```python
from build123d import *

# Parameters (mm, degrees)
EXTRUDE_1_DEPTH     = 12
EXTRUDE_3_DEPTH     = 6
SKETCH_4_R          = 2
EXTRUDE_4_DEPTH     = 4
CUT_EXTRUDE_2_DEPTH = 29.284271247


with BuildPart() as part:
    # 草图1 → 凸台-拉伸1 (new body)
    with BuildSketch(Plane.XY):
        Polygon((-11, 12.536842105), (-16, 12.536842105), (-16, 14.536842105), (-11, 14.536842105), (-11, 16.036842105), (11, 16.036842105), (11, 14.536842105), (16, 14.536842105), (16, 12.536842105), (11, 12.536842105), (11, -5.463157895), (-11, -5.463157895), align=None)
    extrude(amount=EXTRUDE_1_DEPTH)

    # 草图2 → 凸台-拉伸3 (add)
    with BuildSketch(Plane(origin=(0, 16.036842105, 0), x_dir=(1, 0, 0), z_dir=(0, 1, 0))):
        with BuildLine():
            ThreePointArc((-0.479166667, -8.445144707), (11, -6), (-0.479166667, -3.554855293))
            ThreePointArc((-0.479166667, -3.554855293), (-3.5, -6), (-0.479166667, -8.445144707))
        make_face()
    extrude(amount=EXTRUDE_3_DEPTH)

    # 草图4 → 凸台-拉伸4 (add)
    with BuildSketch(Plane(origin=(0, 22.036842105, 0), x_dir=(1, 0, 0), z_dir=(0, 1, 0))):
        with Locations(Location((5, -6, 0), (0, 0, 180))):
            Circle(SKETCH_4_R)
    extrude(amount=EXTRUDE_4_DEPTH)

    # 草图5 → 切除-拉伸2 (cut, through all)
    with BuildSketch(Plane(origin=(0, 14.536842105, 0), x_dir=(-1, 0, 0), z_dir=(0, -1, 0))):
        with BuildLine():
            Line((-14.366025404, -6.458256145), (-16, -6.458256145))
            Line((-16, -6.458256145), (-16, -5.458256145))
            Line((-16, -5.458256145), (-14.366025404, -5.458256145))
            ThreePointArc((-14.366025404, -5.458256145), (-12.5, -5.958256145), (-14.366025404, -6.458256145))
        make_face()
        with BuildLine():
            Line((16, -6.458256145), (16, -5.458256145))
            Line((16, -5.458256145), (14.366025404, -5.458256145))
            ThreePointArc((14.366025404, -5.458256145), (12.5, -5.958256145), (14.366025404, -6.458256145))
            Line((14.366025404, -6.458256145), (16, -6.458256145))
        make_face()
    extrude(amount=CUT_EXTRUDE_2_DEPTH, mode=Mode.SUBTRACT)


solid = part.part
```
Verification items for the finished model (mm, model axes). A direction names the side the tool comes from. Round coordinates to 2 decimals unless told otherwise and drop trailing zeros. Order: outer loops, then holes, each group sorted by start corner. A loop starts at its lowest first (then second) coordinate and runs counter-clockwise, first axis right, second up. Notation, with made-up numbers: (-9.5, 51.25) -> (9.5, 51.25) arc R25 cw to (9.5, 69.25) -> close; hole circle Ø2 at (-25.5, 85.25). An arc over 180 degrees is marked (long way). Put each result on its own line as item: value. Start each with the question number.
(1) Depth check by flat-ended pin: pin 1 Ø3 at (y, z) = (17.5, 6.5) entering from -X; pin 2 Ø0.8 at (y, z) = (15.5, 7) entering from +X; pin 3 Ø1.5 at (x, z) = (-14, 7.5) entering from -Y. Enter the tip coordinate at first touch or a pass-through.
(2) Section check A-A (x = -13.5). Enter the section's corners in (y, z).
(3) Section check D-D (z = 3). Enter the section's corners in (x, y).
(4) Draft check along Z on faces 1 (the face through (-16, 14, 3)), 2 (the face through (15, 14, 5.458)), 3 (the face through (-3.5, 19, 5.9)). Enter one of: +Z half, -Z half, draft (parallel to the pull), parting line (faces both ways), or undercut.
(5) Section check B-B (x = -1). Enter the section's corners in (y, z).
(6) Material ranges on line 1 along X through (y, z) = (14, 6.75); line 2 along X through (y, z) = (0, 0.5); line 3 along Y through (x, z) = (-10, 9), recorded low to high.
(7) Section check C-C (y = 6). Enter the section's corners in (x, z), then the cut area to 3 significant figures.
(8) Tool access check on faces 4 (the face through (-11, 15, 6)), 5 (the face through (-11, 3, 6)), 6 (the face through (-15, 14, 5.458)), 7 (the face through (10, 16.037, 1)), 8 (the face through (12, 14.537, 6)). Record the directions out of +Z, -Z, +X, -X, +Y, -Y that give a thin tool (end or side, any length) a straight path to the whole face; none if there is none.
Completed:
1. pin 1: stops at x = -11
1. pin 2: stops at x = 11
1. pin 3: stops at y = 12.54
2. outline: (12.54, 0) -> (14.54, 0) -> (14.54, 4.96) -> (12.54, 4.96) -> close; (12.54, 6.96) -> (14.54, 6.96) -> (14.54, 12) -> (12.54, 12) -> close
3. outline: (-16, 12.54) -> (-11, 12.54) -> (-11, -5.46) -> (11, -5.46) -> (11, 12.54) -> (16, 12.54) -> (16, 14.54) -> (11, 14.54) -> (11, 16.04) -> (10.2, 16.04) -> (10.2, 22.04) -> (-0.2, 22.04) -> (-0.2, 16.04) -> (-11, 16.04) -> (-11, 14.54) -> (-16, 14.54) -> close
4. face 1: draft
4. face 2: undercut
4. face 3: parting line
5. outline: (-5.46, 0) -> (16.04, 0) -> (16.04, 3.5) -> (22.04, 3.5) -> (22.04, 8.5) -> (16.04, 8.5) -> (16.04, 12) -> (-5.46, 12) -> close
6. line 1: x = -16 to -14.11, -12.89 to 12.89, 14.11 to 16
6. line 2: x = -11 to 11
6. line 3: y = -5.46 to 16.04
7. outline: (-11, 0) -> (11, 0) -> (11, 12) -> (-11, 12) -> close
7. area: 264 mm2
8. face 4: +Z, -Z, -X, +Y
8. face 5: +Z, -Z, -X, -Y
8. face 6: -X, +Y, -Y
8. face 7: -Z, +X, +Y
8. face 8: +Z, -Z, +X, +Y
